Can you work these out from the model? Positions are in its coordinate system, mm. Face numbers are marked on the shaded views. Round coordinates to 2 decimals unless told otherwise and drop trailing zeros. Loops run counter-clockwise (first coordinate to the right, second up) from the corner with the lowest first, then second, coordinate; pieces in that order, holes last. Notation, with made-up numbers: M 15.25,10 L 65.25,10 A18 ccw 65.25,22 Z; hole C 26,-29 d8. An arc over 180 degrees is marked long. Answer as CSV lines item,"result".
from build123d import *

# Parameters (mm, degrees)
CYLINDER003_R     = 1.5
CYLINDER003_DEPTH = 1
CYLINDER001_R     = 4
CYLINDER001_DEPTH = 10
CYLINDER_R        = 5
CYLINDER_DEPTH    = 1
CYLINDER002_R     = 1.5
CYLINDER002_DEPTH = 1


with BuildPart() as cylinder003:
    # Cylinder003 → Cylinder003 (new body)
    with BuildSketch(Plane(origin=(1.5, 5.5, 0), x_dir=(1, 0, 0), z_dir=(0, 0, 1))):
        Circle(CYLINDER003_R)
    extrude(amount=CYLINDER003_DEPTH)


with BuildPart() as cylinder001:
    # Cylinder001 → Cylinder001 (new body)
    with BuildSketch(Plane.XY.offset(-5)):
        Circle(CYLINDER001_R)
    extrude(amount=CYLINDER001_DEPTH)


with BuildPart() as cut:
    # Cylinder → Cylinder (new body)
    with BuildSketch(Plane.XY):
        Circle(CYLINDER_R)
    extrude(amount=CYLINDER_DEPTH)

    # Cut: cut Cylinder001
    add(cylinder001.part, mode=Mode.SUBTRACT)


with BuildPart() as fusion:
    # Cylinder002 → Cylinder002 (new body)
    with BuildSketch(Plane(origin=(-5.5, 2, 0), x_dir=(1, 0, 0), z_dir=(0, 0, 1))):
        Circle(CYLINDER002_R)
    extrude(amount=CYLINDER002_DEPTH)

    # Fusion: union Cylinder003, Cut
    add(cylinder003.part)
    add(cut.part)


solid = fusion.part
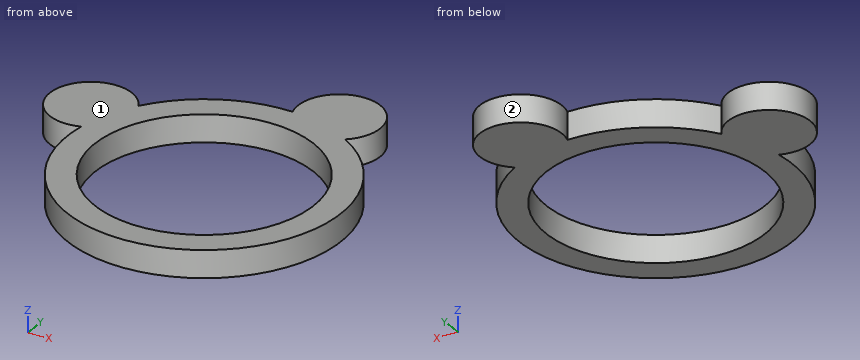
Item 1: If we section it at A-A on y = 0: Write out the boundary of the cut face in (x, z), then the cut area to 3 significant figures.
Output:
outline,"M -5,0 L -4,0 L -4,1 L -5,1 Z; M 4,0 L 5,0 L 5,1 L 4,1 Z"
area,"2.00 mm2"
Item 2: If we section it at D-D on y = 5.5: Write out the boundary of the cut face in (x, z).
Output:
outline,"M 0,0 L 3,0 L 3,1 L 0,1 Z"
Item 3: If we section it at B-B on x = 1.5: Write out the boundary of the cut face in (y, z).
Output:
outline,"M -4.77,0 L -3.71,0 L -3.71,1 L -4.77,1 Z; M 3.71,0 L 7,0 L 7,1 L 3.71,1 Z"
Item 4: If we section it at C-C on z = 0.85: Write out the boundary of the cut face in (x, y).
Output:
outline,"M -4.96,0.6 A5 ccw long 2.46,4.35 A1.5 ccw long 0.09,5 A5 ccw -4.19,2.73 A1.5 ccw long Z; hole C 0,0 d8"
Item 5: We'd pull the mould along Y, two halves only. Please class the marked faces 1 and 2: released by +Y, released by -Y, zero draft, split by the parting line, or undercut.
Output:
face 1,"zero draft"
face 2,"undercut"
Item 6: If I drill on line 1 along X through (y, z) = (0, 0.8); line 2 along Y through (x, z) = (2.75, 0.85); line 3 along Y through (x, z) = (-3.5, 0.6), over which ranges is the centre line in solid material (lowest first)? Write a range as from..to.
Output:
line 1,"x = -5..-4, 4..5"
line 2,"y = -4.18..-2.9, 2.9..4.18, 4.67..6.33"
line 3,"y = -3.57..-1.94, 1.94..3.57"
